The figure shows three views and two pictorial views of one solid part (mm, origin at its lowest corner). Answer the questions. Coordinates: 2 decimals unless noted, no trailing zeros. Write each loop counter-clockwise with the first axis right and the second up, starting at its lowest first coordinate (ties: lowest second). Pieces come first, ordered by that corner, then holes.
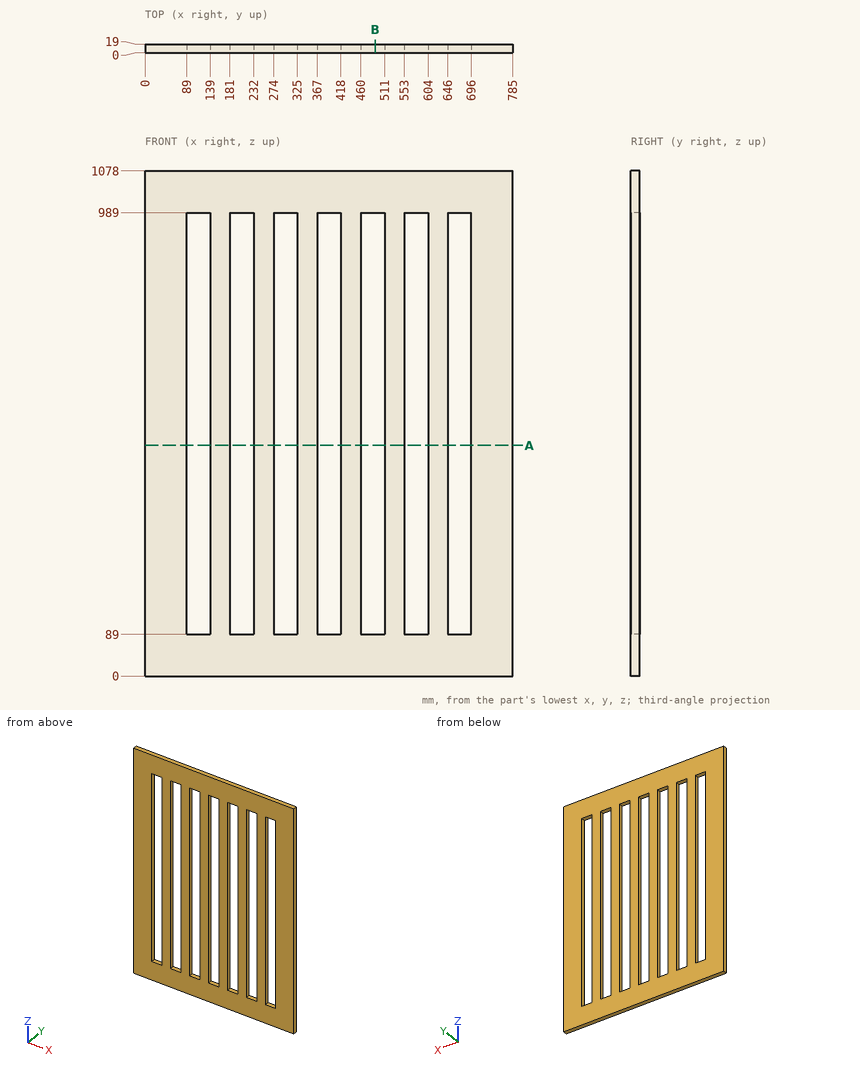
1. Find the intervals of material crossed by L1, parallel to Z at x = 383, y = 8, in increasing order.
Results found:
L1: z = 0 to 89, 989 to 1078
2. A flat-ended cylindrical pin translates along its axis: P1, Ø9.5, axis at y = 10.5, z = 724, coming from the -X side. Find the tip coordinate at first contact, or state that the pin passes through.
Results found:
P1: stops at x = 0
3. Section B-B on x = 491 is taken. Give the vertices of the cut face in (y, z), then the cut area to 3 significant figures.
Results found:
outline: (0, 0) - (19, 0) - (19, 89) - (0, 89) - close; (0, 989) - (19, 989) - (19, 1078) - (0, 1078) - close
area: 3,380 mm2
4. Section A-A on z = 492 is taken. State how many separate pieces and enclosed holes the cut face has, then the cut area to 3 significant figures.
Results found:
separate pieces: 8
enclosed holes: 0
area: 8,170 mm2
